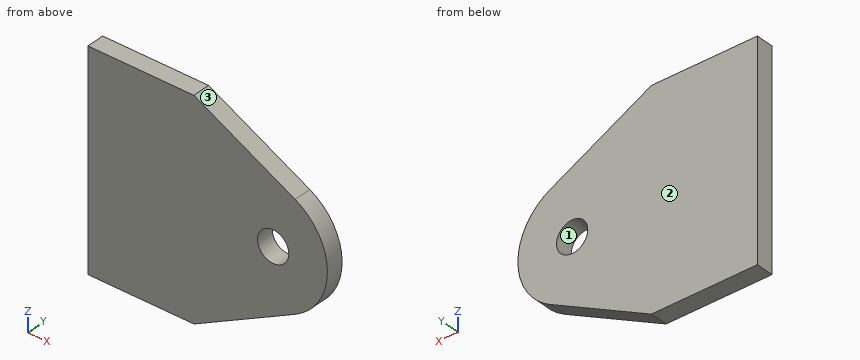
from build123d import *

# Parameters (mm, degrees)
F1_DEPTH = 12.7
F2_D     = 22.479


with BuildPart() as f1:
    # F0 (on Front) → F1 (new body)
    with BuildSketch(Plane.XZ):
        with BuildLine():
            Line((-35.987624, 76.2), (-112.187624, 76.2))
            Line((-112.187624, 76.2), (-112.187624, -76.2))
            Line((-112.187624, -76.2), (-35.987624, -76.2))
            Line((-35.987624, -76.2), (36.712844, -38.322777))
            ThreePointArc((36.712844, -38.322777), (59.958668, 0), (36.712844, 38.322777))
            Line((36.712844, 38.322777), (-35.987624, 76.2))
        make_face()
    extrude(amount=F1_DEPTH)

    # F2 (through all)
    with Locations(Plane(origin=(0, 0, 0), x_dir=(1, 0, 0), z_dir=(0, 1, 0))):
        with Locations((20.97105, 0)):
            Hole(F2_D / 2)


solid = f1.part
The listing builds one solid part. Answer for the finished solid, in the listing's coordinates (mm). Face numbers are marked on the shaded views. Give positions to 0.01 mm unless a question says otherwise; leave off trailing zeros. Write each loop counter-clockwise with the first axis right and the second up, starting at its lowest first coordinate (ties: lowest second). Pieces come first, ordered by that corner, then holes.
Item 1: Section B-B, the plane y = -7.25 is taken. Write down the section's boundary in (x, z).
Item 2: A flat-ended cylindrical pin translates along its axis: P1, Ø3, axis at y = -9, z = -10.5, coming from the +X side. Find the tip coordinate at first contact, or state that the pin passes through.
Item 3: Section A-A, the plane z = 0 is taken. Write down the section's boundary in (x, y), plus the area to 3 significant figures.
Item 4: Find the intervals of material crossed by line 1 along X through (y, z) = (-10.75, 9.5); line 2 along X through (y, z) = (-6.5, -6); line 3 along Z through (x, y) = (13, -11.25), in increasing order.
Item 5: Section D-D, the plane z = -27 is taken. Write down the section's boundary in (x, y).
Item 6: Section C-C, the plane x = 45.5 is taken. Write down the section's boundary in (y, z), plus the area to 3 significant figures.
Item 7: Determine the mould class of the marked faces 1, 2 and 3 for opening direction Z: released by +Z, released by -Z, zero draft, split by the parting line, or undercut.
Completed:
1. outline: (-112.19, -76.2) - (-35.99, -76.2) - (36.71, -38.32) arc R43.21 ccw to (36.71, 38.32) - (-35.99, 76.2) - (-112.19, 76.2) - close; hole circle Ø22.48 at (20.97, 0)
2. P1: stops at x = 59.01
3. outline: (-112.19, -12.7) - (9.73, -12.7) - (9.73, 0) - (-112.19, 0) - close; (32.21, -12.7) - (59.96, -12.7) - (59.96, 0) - (32.21, 0) - close
3. area: 1,900 mm2
4. line 1: x = -112.19 to 14.96, 26.98 to 58.9
4. line 2: x = -112.19 to 11.47, 30.48 to 59.54
4. line 3: z = -50.68 to -7.92, 7.92 to 50.68
5. outline: (-112.19, -12.7) - (50.49, -12.7) - (50.49, 0) - (-112.19, 0) - close
6. outline: (-12.7, -32.26) - (0, -32.26) - (0, 32.26) - (-12.7, 32.26) - close
6. area: 819 mm2
7. face 1: undercut
7. face 2: zero draft
7. face 3: released by +Z
